Read the model definition and answer for the solid it produces. Units are mm, in the model's axes. A direction names the side the tool comes from. Give positions to 0.01 mm unless a question says otherwise; leave off trailing zeros. Write each loop counter-clockwise with the first axis right and the second up, starting at its lowest first coordinate (ties: lowest second). Pieces come first, ordered by that corner, then holes.
```python
from build123d import *

# Parameters (mm, degrees)
SKETCH1_R               = 1
BOSS_EXTRUDE1_DEPTH     = 2
SKETCH2_R               = 9.5
SKETCH2_R_2             = 1
SKETCH2_R_3             = 2.25
BOSS_EXTRUDE2_DEPTH     = 15
CUT_EXTRUDE1_DEPTH      = 13
CUT_EXTRUDE1_DEPTH_BACK = 31.1579177
SKETCH2_3_R             = 9.5
SKETCH2_3_R_2           = 2.25
CHAMFER1_SIZE           = 2
FILLET1_R               = 2


with BuildPart() as part:
    # Sketch1 → Boss-Extrude1 (new body)
    with BuildSketch(Plane.XY.offset(3)):
        with BuildLine():
            ThreePointArc((-3.861100009, -18.092592593), (0, -18.5), (3.861100009, -18.092592593))
            ThreePointArc((3.861100009, -18.092592593), (5.499959243, -15.898009243), (5.992679576, -13.203703704))
            ThreePointArc((5.992679576, -13.203703704), (10.253048327, -10.253048327), (13.203703704, -5.992679576))
            ThreePointArc((13.203703704, -5.992679576), (15.898009243, -5.499959243), (18.092592593, -3.861100009))
            ThreePointArc((18.092592593, -3.861100009), (18.5, 0), (18.092592593, 3.861100009))
            ThreePointArc((18.092592593, 3.861100009), (15.898009243, 5.499959243), (13.203703704, 5.992679576))
            ThreePointArc((13.203703704, 5.992679576), (10.253048327, 10.253048327), (5.992679576, 13.203703704))
            ThreePointArc((5.992679576, 13.203703704), (5.499959243, 15.898009243), (3.861100009, 18.092592593))
            ThreePointArc((3.861100009, 18.092592593), (0, 18.5), (-3.861100009, 18.092592593))
            ThreePointArc((-3.861100009, 18.092592593), (-5.499959243, 15.898009243), (-5.992679576, 13.203703704))
            ThreePointArc((-5.992679576, 13.203703704), (-10.253048327, 10.253048327), (-13.203703704, 5.992679576))
            ThreePointArc((-13.203703704, 5.992679576), (-15.898009243, 5.499959243), (-18.092592593, 3.861100009))
            ThreePointArc((-18.092592593, 3.861100009), (-18.5, 0), (-18.092592593, -3.861100009))
            ThreePointArc((-18.092592593, -3.861100009), (-15.898009243, -5.499959243), (-13.203703704, -5.992679576))
            ThreePointArc((-13.203703704, -5.992679576), (-10.253048327, -10.253048327), (-5.992679576, -13.203703704))
            ThreePointArc((-5.992679576, -13.203703704), (-5.499959243, -15.898009243), (-3.861100009, -18.092592593))
        make_face()
        with Locations((13.5, 0)):
            Circle(SKETCH1_R, mode=Mode.SUBTRACT)
        with Locations((0, 13.5)):
            Circle(SKETCH1_R, mode=Mode.SUBTRACT)
        with Locations((-13.5, 0)):
            Circle(SKETCH1_R, mode=Mode.SUBTRACT)
        with Locations((0, -13.5)):
            Circle(SKETCH1_R, mode=Mode.SUBTRACT)
    extrude(amount=BOSS_EXTRUDE1_DEPTH)

    # Sketch2 → Boss-Extrude2 (add)
    # profile 1 of 2: a face of its own
    with BuildSketch(Plane.XY.offset(5)):
        with BuildLine():
            ThreePointArc((2.978187161, 13.861111111), (3.800103213, 11.661877619), (5.535216541, 10.080246914))
            ThreePointArc((5.535216541, 10.080246914), (8.131727984, 8.131727984), (10.080246914, 5.535216541))
            ThreePointArc((10.080246914, 5.535216541), (11.661877619, 3.800103213), (13.861111111, 2.978187161))
            ThreePointArc((13.861111111, 2.978187161), (16.5, 0), (13.861111111, -2.978187161))
            ThreePointArc((13.861111111, -2.978187161), (11.661877619, -3.800103213), (10.080246914, -5.535216541))
            ThreePointArc((10.080246914, -5.535216541), (8.131727984, -8.131727984), (5.535216541, -10.080246914))
            ThreePointArc((5.535216541, -10.080246914), (3.800103213, -11.661877619), (2.978187161, -13.861111111))
            ThreePointArc((2.978187161, -13.861111111), (0, -16.5), (-2.978187161, -13.861111111))
            ThreePointArc((-2.978187161, -13.861111111), (-3.800103213, -11.661877619), (-5.535216541, -10.080246914))
            ThreePointArc((-5.535216541, -10.080246914), (-8.131727984, -8.131727984), (-10.080246914, -5.535216541))
            ThreePointArc((-10.080246914, -5.535216541), (-11.661877619, -3.800103213), (-13.861111111, -2.978187161))
            ThreePointArc((-13.861111111, -2.978187161), (-16.5, 0), (-13.861111111, 2.978187161))
            ThreePointArc((-13.861111111, 2.978187161), (-11.661877619, 3.800103213), (-10.080246914, 5.535216541))
            ThreePointArc((-10.080246914, 5.535216541), (-8.131727984, 8.131727984), (-5.535216541, 10.080246914))
            ThreePointArc((-5.535216541, 10.080246914), (-3.800103213, 11.661877619), (-2.978187161, 13.861111111))
            ThreePointArc((-2.978187161, 13.861111111), (0, 16.5), (2.978187161, 13.861111111))
        make_face()
        Circle(SKETCH2_R, mode=Mode.SUBTRACT)
        with Locations((-13.5, 0)):
            Circle(SKETCH2_R_2, mode=Mode.SUBTRACT)
        with Locations((13.5, 0)):
            Circle(SKETCH2_R_2, mode=Mode.SUBTRACT)
        with Locations((0, 13.5)):
            Circle(SKETCH2_R_2, mode=Mode.SUBTRACT)
        with Locations((0, -13.5)):
            Circle(SKETCH2_R_2, mode=Mode.SUBTRACT)
    # profile 2 of 2: a face of its own
    with BuildSketch(Plane.XY.offset(5)):
        Circle(SKETCH2_R)
        Circle(SKETCH2_R_3, mode=Mode.SUBTRACT)
    extrude(amount=BOSS_EXTRUDE2_DEPTH)

    # Sketch2<3> → Cut-Extrude1 (cut, two sides: drawn at the far end of the back side and taken through both)
    # profile 1 of 2: a face of its own
    with BuildSketch(Plane.XY.offset(5).offset(-CUT_EXTRUDE1_DEPTH_BACK)):
        Circle(SKETCH2_3_R)
        Circle(SKETCH2_3_R_2, mode=Mode.SUBTRACT)
    # profile 2 of 2: a face of its own
    with BuildSketch(Plane.XY.offset(5).offset(-CUT_EXTRUDE1_DEPTH_BACK)):
        Circle(SKETCH2_3_R_2)
    extrude(amount=CUT_EXTRUDE1_DEPTH + CUT_EXTRUDE1_DEPTH_BACK, mode=Mode.SUBTRACT)

    # Chamfer1
    chamfer1_edges = [part.edges().sort_by_distance(p)[0] for p in [
        (-9.5, 0, 3),
    ]]
    chamfer(chamfer1_edges, length=CHAMFER1_SIZE - 0.0001)  # a hair under: the kernel refuses the full size

    # Fillet1
    fillet1_edges = [part.edges().sort_by_distance(p)[0] for p in [
        (-16.5, 0, 5),
        (-11.661877619, -3.800103213, 5),
        (-8.131727984, -8.131727984, 5),
        (0, -16.5, 5),
        (3.800103213, -11.661877619, 5),
        (8.131727984, -8.131727984, 5),
        (16.5, 0, 5),
        (11.661877619, 3.800103213, 5),
        (8.131727984, 8.131727984, 5),
        (3.800103213, 11.661877619, 5),
        (11.661877619, -3.800103213, 5),
        (-3.800103213, -11.661877619, 5),
        (-11.661877619, 3.800103213, 5),
        (0, 16.5, 5),
        (-3.800103213, 11.661877619, 5),
        (-8.131727984, 8.131727984, 5),
    ]]
    fillet(fillet1_edges, radius=FILLET1_R - 0.0001)  # a hair under: the kernel refuses the full size


solid = part.part
```
Item 1: Section A-A (x = 0) is taken. Give the number of separate pieces and of enclosed holes in the cut face, and give its area (3 significant figures).
Result set:
separate pieces: 4
enclosed holes: 0
area: 205 mm2
Item 2: Find the intervals of material crossed by line 1 along Y through (x, z) = (0, 10.25); line 2 along Z through (x, y) = (4, -4); line 3 along X through (y, z) = (2, 15.5), in increasing order.
Result set:
line 1: y = -16.5 to -14.5, -12.5 to -9.5, 9.5 to 12.5, 14.5 to 16.5
line 2: z = 18 to 20
line 3: x = -15.74 to -9.29, 9.29 to 15.74
Item 3: Each of these flat-tipped pins is pushed along its axis until it touches: pin 1 Ø9.5 at (x, y) = (-3.5, -1.5) entering from -Z; pin 2 Ø3 at (x, y) = (-6, -9) entering from -Z; pin 3 Ø1.5 at (x, z) = (10, 11.5) entering from +Y; pin 4 Ø1.6 at (x, y) = (-13.5, 0) entering from -Z. Where does it stop, or does it pass through?
Result set:
pin 1: stops at z = 18
pin 2: stops at z = 3
pin 3: stops at y = 6.83
pin 4: passes through
Item 4: Determine the mould class of faces 1 (the cylindrical face through (3.82, -11.63, 13.41)), 2 (the cylindrical face through (-0.29, 2.23, 18.99)), 3 (the cylindrical face through (-0.217, -14.476, 11.381)), 4 (the cylindrical face through (-18.5, 0.1, 4)) for opening direction X: pulls with the +X half, pulls with the -X half, needs draft (parallel to the pull), parting line crosses it, or undercut.
Result set:
face 1: pulls with the +X half
face 2: undercut
face 3: undercut
face 4: pulls with the -X half
Item 5: Section C-C (z = 8.75) is taken. Write down the section's boundary in (x, y), and give its area (3 significant figures).
Result set:
outline: (-13.86, -2.98) arc R5 cw to (-10.08, -5.54) arc R11.5 ccw to (-5.54, -10.08) arc R5 cw to (-2.98, -13.86) arc R3 ccw to (2.98, -13.86) arc R5 cw to (5.54, -10.08) arc R11.5 ccw to (10.08, -5.54) arc R5 cw to (13.86, -2.98) arc R3 ccw to (13.86, 2.98) arc R5 cw to (10.08, 5.54) arc R11.5 ccw to (5.54, 10.08) arc R5 cw to (2.98, 13.86) arc R3 ccw to (-2.98, 13.86) arc R5 cw to (-5.54, 10.08) arc R11.5 ccw to (-10.08, 5.54) arc R5 cw to (-13.86, 2.98) arc R3 ccw to start; hole circle Ø2 at (-13.5, 0); hole circle Ø19 at (0, 0); hole circle Ø2 at (0, -13.5); hole circle Ø2 at (0, 13.5); hole circle Ø2 at (13.5, 0)
area: 240 mm2
Item 6: Which of the six approach directions +Z, -Z, +X, -X, +Y, -Y give full straight-line access (tool end or side, diameter ignored) to faces 5 (the cylindrical face through (-0.1, 16.5, 13.4)), 6 (the flat face through (-10, 10, 5)), 7 (the flat face through (2, -2, 18)), 8 (the cylindrical face through (-11.63, -3.82, 13.41))?
Result set:
face 5: +Z, +Y
face 6: +Z
face 7: -Z
face 8: +Z, -X, -Y
